Verification items for this drawing (mm, ordinates from the low corner). A direction names the side the tool comes from. Round coordinates to 2 decimals unless told otherwise and drop trailing zeros. Order: outer loops, then holes, each group sorted by start corner. A loop starts at its lowest first (then second) coordinate and runs counter-clockwise, first axis right, second up. Notation, with made-up numbers: M 3.25,89.25 L 21.25,89.25 A21 cw 21.25,108.25 Z; hole C -4,20.25 d1. An arc over 180 degrees is marked long. Use CSV: the item, a comma, the result in double quotes. Start each with the question number.
Q1. Scan lines: line 1 (Y direction, x = 4.5, z = 18.05); line 2 (X direction, y = 12, z = 9.75); line 3 (Z direction, x = 11.5, y = 47). Record each from-to range of solid material in increasing order.
Q2. Set-up check for the marked faces 1, 2, 3, 4 and 5: record each of +Z, -Z, +X, -X, +Y, -Y from which the full face is reachable in a straight line by a thin tool's end or side.
Q3. Mould release check, pull along Z, two halves, no side actions. Record for the marked faces 6, 7 and 8: +Z half, -Z half, draft (parallel to the pull), parting line (faces both ways), or undercut.
Q4. Gauge pin test, flat ends, axial feed: pin 1 Ø10 at (y, z) = (9, 13) entering from -X; pin 2 Ø2.5 at (x, z) = (11, 11) entering from -Y; pin 3 Ø3.5 at (x, z) = (10, 9.5) entering from +Y. Record the tip position at first contact, or that the pin passes through.
Q5. Sectioned sample at A-A (y = 31.5). Enter the section's corners in (x, z).
Q6. Sectioned sample at C-C (z = 10.5). Enter the section's corners in (x, y), and give its area (3 significant figures).
Q7. Sectioned sample at B-B (x = 10.25). Enter the section's corners in (y, z), and give its area (3 significant figures).
Q8. Sectioned sample at D-D (x = 3.5). Enter the section's corners in (y, z), and give its area (3 significant figures).
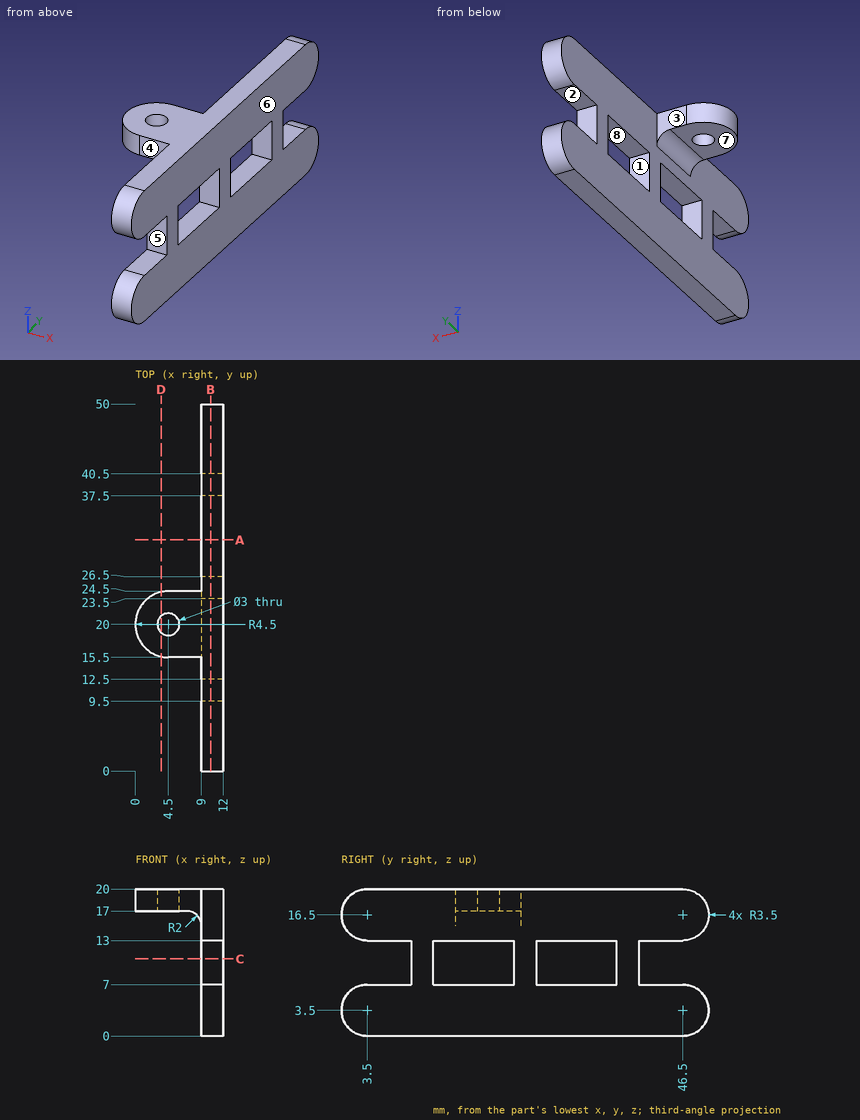
Verdict:
1,line 1,"y = 15.5 to 18.5, 21.5 to 24.5"
1,line 2,"x = 9 to 12"
1,line 3,"z = 0.04 to 6.96, 13.04 to 19.96"
2,face 1,"+X, -X"
2,face 2,"+X, -X, +Y"
2,face 3,"+Z, -Z, -X, +Y"
2,face 4,"+Z, -Z, -X, -Y"
2,face 5,"+X, -X, -Y"
3,face 6,"draft"
3,face 7,"-Z half"
3,face 8,"undercut"
4,pin 1,"stops at x = 9"
4,pin 2,"stops at y = 9.5"
4,pin 3,"stops at y = 40.5"
5,outline,"M 9,0 L 12,0 L 12,7 L 9,7 Z; M 9,13 L 12,13 L 12,20 L 9,20 Z"
6,outline,"M 9,9.5 L 12,9.5 L 12,12.5 L 9,12.5 Z; M 9,23.5 L 12,23.5 L 12,26.5 L 9,26.5 Z; M 9,37.5 L 12,37.5 L 12,40.5 L 9,40.5 Z"
6,area,"27.0 mm²"
7,outline,"M 3.5,0 L 46.5,0 A3.5 ccw 46.5,7 L 40.5,7 L 40.5,13 L 46.5,13 A3.5 ccw 46.5,20 L 3.5,20 A3.5 ccw 3.5,13 L 9.5,13 L 9.5,7 L 3.5,7 A3.5 ccw Z; hole M 12.5,7 L 23.5,7 L 23.5,13 L 12.5,13 Z; hole M 26.5,7 L 37.5,7 L 37.5,13 L 26.5,13 Z"
7,area,"733 mm²"
8,outline,"M 15.61,17 L 18.88,17 L 18.88,20 L 15.61,20 Z; M 21.12,17 L 24.39,17 L 24.39,20 L 21.12,20 Z"
8,area,"19.6 mm²"
